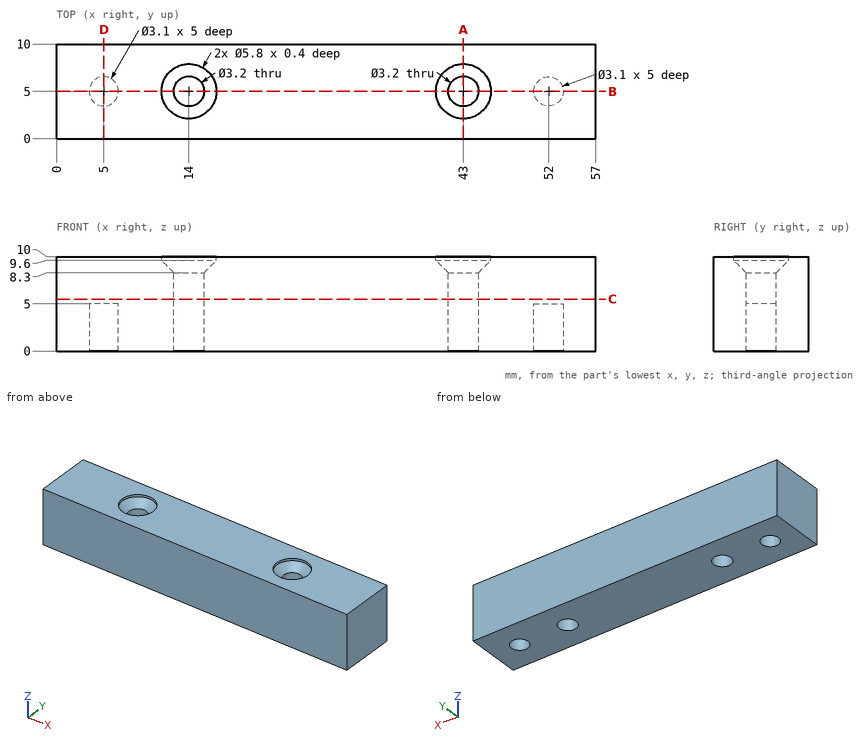
Print and shaded views of the part. All mm, measured from the part's lowest x, y and z. Give positions to 0.01 mm unless a question says otherwise; leave off trailing zeros. Loops run counter-clockwise (first coordinate to the right, second up) from the corner with the lowest first, then second, coordinate; pieces in that order, holes last.
1) Saw through at C-C (z = 5.5). Write the cut outline in (x, y).
2) Saw through at A-A (x = 43). Write the cut outline in (y, z), plus the area to 3 significant figures.
3) Wall check: line 1 (X direction, y = 5, z = 9.9); line 2 (Y direction, x = 14, z = 9.7); line 3 (X direction, y = 6, z = 7.5). Give the ranges that are in metal, low to high.
4) Saw through at B-B (y = 5). Write the cut outline in (x, z), plus the area to 3 significant figures.
5) Saw through at D-D (x = 5). Write the cut outline in (y, z), plus the area to 3 significant figures.
6) Flat gauge pins, fed straight in: pin 1 Ø4.5 at (x, y) = (14, 5) entering from +Z; pin 2 Ø3 at (x, y) = (43, 5) entering from +Z; pin 3 Ø0.9 at (x, y) = (4.5, 5) entering from -Z. Where does each tip first touch, or does it go through?
Answer block:
1. outline: (0, 0) - (57, 0) - (57, 10) - (0, 10) - close; hole circle Ø3.2 at (14, 5); hole circle Ø3.2 at (43, 5)
2. outline: (0, 0) - (3.4, 0) - (3.4, 8.3) - (2.1, 9.6) - (2.1, 10) - (0, 10) - close; (6.6, 0) - (10, 0) - (10, 10) - (7.9, 10) - (7.9, 9.6) - (6.6, 8.3) - close
2. area: 65.3 mm2
3. line 1: x = 0 to 11.1, 16.9 to 40.1, 45.9 to 57
3. line 2: y = 0 to 2.1, 7.9 to 10
3. line 3: x = 0 to 12.75, 15.25 to 41.75, 44.25 to 57
4. outline: (0, 0) - (3.45, 0) - (3.45, 5) - (6.55, 5) - (6.55, 0) - (12.4, 0) - (12.4, 8.3) - (11.1, 9.6) - (11.1, 10) - (0, 10) - close; (15.6, 0) - (41.4, 0) - (41.4, 8.3) - (40.1, 9.6) - (40.1, 10) - (16.9, 10) - (16.9, 9.6) - (15.6, 8.3) - close; (44.6, 0) - (50.45, 0) - (50.45, 5) - (53.55, 5) - (53.55, 0) - (57, 0) - (57, 10) - (45.9, 10) - (45.9, 9.6) - (44.6, 8.3) - close
4. area: 470 mm2
5. outline: (0, 0) - (3.45, 0) - (3.45, 5) - (6.55, 5) - (6.55, 0) - (10, 0) - (10, 10) - (0, 10) - close
5. area: 84.5 mm2
6. pin 1: stops at z = 8.95
6. pin 2: passes through
6. pin 3: stops at z = 5
